```python
from build123d import *

# Parameters (mm, degrees)
SKETCH_1_W          = 47
SKETCH_1_H          = 9
EXTRUDE_1_DEPTH     = 6.5
SKETCH_2_R          = 3
EXTRUDE_2_DEPTH     = 3.5
SKETCH_3_R          = 3.5
EXTRUDE_3_DEPTH     = 0.5
SKETCH_4_R          = 1.65
CUT_EXTRUDE_1_DEPTH = 10
SKETCH_5_R          = 1.65
CUT_EXTRUDE_2_DEPTH = 9
FILLET_1_R          = 1


with BuildPart() as part:
    # ｽｹｯﾁ1 → ﾎﾞｽ - 押し出し1 (new body)
    with BuildSketch(Plane.XY):
        with Locations((23.5, 4.5)):
            Rectangle(SKETCH_1_W, SKETCH_1_H)
    extrude(amount=EXTRUDE_1_DEPTH)

    # ｽｹｯﾁ2 → ﾎﾞｽ - 押し出し2 (add)
    with BuildSketch(Plane.XY.offset(6.5)):
        with Locations(Location((5.5, 5, 0), (0, 0, 180))):
            Circle(SKETCH_2_R)
        with Locations(Location((17.5, 5, 0), (0, 0, 180))):
            Circle(SKETCH_2_R)
        with Locations(Location((29.5, 5, 0), (0, 0, 180))):
            Circle(SKETCH_2_R)
        with Locations(Location((41.5, 5, 0), (0, 0, 180))):
            Circle(SKETCH_2_R)
    extrude(amount=EXTRUDE_2_DEPTH)

    # ｽｹｯﾁ3 → ﾎﾞｽ - 押し出し3 (add)
    with BuildSketch(Plane.XY.offset(6.5)):
        with Locations(Location((5.5, 5, 0), (0, 0, 180))):
            Circle(SKETCH_3_R)
        with Locations(Location((17.5, 5, 0), (0, 0, 180))):
            Circle(SKETCH_3_R)
        with Locations(Location((29.5, 5, 0), (0, 0, 180))):
            Circle(SKETCH_3_R)
        with Locations(Location((41.5, 5, 0), (0, 0, 180))):
            Circle(SKETCH_3_R)
    extrude(amount=EXTRUDE_3_DEPTH)

    # ｽｹｯﾁ4 → ｶｯﾄ - 押し出し1 (cut)
    with BuildSketch(Plane.XY.offset(10)):
        with Locations((5.5, 5)):
            Circle(SKETCH_4_R)
        with Locations((17.5, 5)):
            Circle(SKETCH_4_R)
        with Locations((29.5, 5)):
            Circle(SKETCH_4_R)
        with Locations((41.5, 5)):
            Circle(SKETCH_4_R)
    extrude(amount=-CUT_EXTRUDE_1_DEPTH, mode=Mode.SUBTRACT)

    # ｽｹｯﾁ5 → ｶｯﾄ - 押し出し2 (cut)
    with BuildSketch(Plane(origin=(0, 9, 0), x_dir=(1, 0, 0), z_dir=(0, 1, 0))):
        with Locations(Location((11, -3.25, 0), (0, 0, 270))):
            Circle(SKETCH_5_R)
        with Locations(Location((36, -3.25, 0), (0, 0, 270))):
            Circle(SKETCH_5_R)
    extrude(amount=-CUT_EXTRUDE_2_DEPTH, mode=Mode.SUBTRACT)

    # ﾌｨﾚｯﾄ1
    fillet_1_edges = [part.edges().sort_by_distance(p)[0] for p in [
        (0, 9, 3.25),
        (47, 9, 3.25),
        (47, 0, 3.25),
        (0, 0, 3.25),
    ]]
    fillet(fillet_1_edges, radius=FILLET_1_R)


solid = part.part
```
The listing builds one solid part. Answer for the finished solid, in the listing's coordinates (mm). A direction names the side the tool comes from. Coordinates: 2 decimals unless noted, no trailing zeros. Write each loop counter-clockwise with the first axis right and the second up, starting at its lowest first coordinate (ties: lowest second). Pieces come first, ordered by that corner, then holes. Notation, with made-up numbers: M 67,-38.5 L 97,-38.5 A15 ccw 97,-14.5 Z; hole C 67,-27 d10. An arc over 180 degrees is marked long. Use a Markdown table: item, result. Add a question column.
1. Which of the six approach directions +Z, -Z, +X, -X, +Y, -Y give full straight-line access (tool end or side, diameter ignored) to faces 1 (the cylindrical face through (28.19, 4, 5.07)), 2 (the cylindrical face through (44.997, 4.846, 6.746))?
2. For a pull along Z with two mould halves and no side action, classify faces 3 (the flat face through (40, 6, 10)), 4 (the cylindrical face through (19.024, 4.368, 5.07)), 5 (the cylindrical face through (37.39, 4.56, 4.14)) as +Z half, -Z half, draft (parallel to the pull), parting line (faces both ways), or undercut.
3. Section D-D (x = 5.5) is taken. Give the vertices of the cut face in (y, z).
4. Section C-C (z = 9) is taken. Give the vertices of the cut face in (x, y).
5. Straight lines are drawn through the part: line 1 along X through (y, z) = (3, 3.25); line 2 along X through (y, z) = (7.5, 7.5); line 3 along Y through (x, z) = (29.5, 6). For each, find the intervals that lie inside material, in ascending order. Write a range as [from, to].
6. Section B-B (x = 11) is taken. Give the vertices of the cut face in (y, z).
7. Section A-A (z = 3.25) is taken. Give the vertices of the cut face in (x, y), plus the area to 3 significant figures.
Data:
| question | item | result |
|---|---|---|
| 1 | face 1 | +Z, -Z |
| 1 | face 2 | +Z |
| 2 | face 3 | +Z half |
| 2 | face 4 | draft |
| 2 | face 5 | undercut |
| 3 | outline | M 0,0 L 3.35,0 L 3.35,10 L 2,10 L 2,7 L 1.5,7 L 1.5,6.5 L 0,6.5 Z; M 6.65,0 L 9,0 L 9,6.5 L 8.5,6.5 L 8.5,7 L 8,7 L 8,10 L 6.65,10 Z |
| 4 | outline | C 5.5,5 d6; C 17.5,5 d6; C 29.5,5 d6; C 41.5,5 d6; hole C 5.5,5 d3.3; hole C 17.5,5 d3.3; hole C 29.5,5 d3.3; hole C 41.5,5 d3.3 |
| 5 | line 1 | x = [0, 9.35], [12.65, 34.35], [37.65, 47] |
| 5 | line 2 | x = [3.84, 7.16], [15.84, 19.16], [27.84, 31.16], [39.84, 43.16] |
| 5 | line 3 | y = [0, 3.35], [6.65, 9] |
| 6 | outline | M 0,0 L 9,0 L 9,1.6 L 0,1.6 Z; M 0,4.9 L 9,4.9 L 9,6.5 L 0,6.5 Z |
| 7 | outline | M 0,1 A1 ccw 1,0 L 9.35,0 L 9.35,9 L 1,9 A1 ccw 0,8 Z; M 12.65,0 L 34.35,0 L 34.35,9 L 12.65,9 Z; M 37.65,0 L 46,0 A1 ccw 47,1 L 47,8 A1 ccw 46,9 L 37.65,9 Z; hole C 5.5,5 d3.3; hole C 17.5,5 d3.3; hole C 29.5,5 d3.3; hole C 41.5,5 d3.3 |
| 7 | area | 329 mm2 |
